from build123d import *

# Parameters (mm, degrees)
SKETCH1_R           = 31.5
SKETCH1_R_2         = 2.6
BOSS_EXTRUDE1_DEPTH = 5
SKETCH2_R           = 12.53
SKETCH2_R_2         = 9.53
BOSS_EXTRUDE2_DEPTH = 15
CUT_EXTRUDE1_START  = -7
CUT_EXTRUDE1_DEPTH  = 7
FILLET1_R           = 5
FILLET2_R           = 2
FILLET3_R           = 2


with BuildPart() as part:
    # Sketch1 → Boss-Extrude1 (new body)
    with BuildSketch(Plane.XY):
        Circle(SKETCH1_R)
        with Locations((0, 25)):
            Circle(SKETCH1_R_2, mode=Mode.SUBTRACT)
        with Locations((25, 0)):
            Circle(SKETCH1_R_2, mode=Mode.SUBTRACT)
        with Locations((0, -25)):
            Circle(SKETCH1_R_2, mode=Mode.SUBTRACT)
        with Locations((-25, 0)):
            Circle(SKETCH1_R_2, mode=Mode.SUBTRACT)
    extrude(amount=BOSS_EXTRUDE1_DEPTH)

    # Sketch2 → Boss-Extrude2 (add)
    with BuildSketch(Plane.XY.offset(5)):
        Circle(SKETCH2_R)
        Circle(SKETCH2_R_2, mode=Mode.SUBTRACT)
    extrude(amount=BOSS_EXTRUDE2_DEPTH)

    # Sketch3 → Cut-Extrude1 (cut)
    with BuildSketch(Plane.XY.offset(5).offset(CUT_EXTRUDE1_START)):
        with BuildLine():
            ThreePointArc((-14.488887394, 3.882285677), (-10.606601718, 10.606601718), (-3.882285677, 14.488887394))
            Line((-3.882285677, 14.488887394), (-8.152799921, 30.426663528))
            ThreePointArc((-8.152799921, 30.426663528), (-22.273863607, 22.273863607), (-30.426663528, 8.152799921))
            Line((-30.426663528, 8.152799921), (-14.488887394, 3.882285677))
        make_face()
        with BuildLine():
            Line((8.152799921, 30.426663528), (3.882285677, 14.488887394))
            ThreePointArc((3.882285677, 14.488887394), (10.606601718, 10.606601718), (14.488887394, 3.882285677))
            Line((14.488887394, 3.882285677), (30.426663528, 8.152799921))
            ThreePointArc((30.426663528, 8.152799921), (22.273863607, 22.273863607), (8.152799921, 30.426663528))
        make_face()
        with BuildLine():
            Line((30.426663528, -8.152799921), (14.488887394, -3.882285677))
            ThreePointArc((14.488887394, -3.882285677), (10.606601718, -10.606601718), (3.882285677, -14.488887394))
            Line((3.882285677, -14.488887394), (8.152799921, -30.426663528))
            ThreePointArc((8.152799921, -30.426663528), (22.273863607, -22.273863607), (30.426663528, -8.152799921))
        make_face()
        with BuildLine():
            Line((-8.152799921, -30.426663528), (-3.882285677, -14.488887394))
            ThreePointArc((-3.882285677, -14.488887394), (-10.606601718, -10.606601718), (-14.488887394, -3.882285677))
            Line((-14.488887394, -3.882285677), (-30.426663528, -8.152799921))
            ThreePointArc((-30.426663528, -8.152799921), (-22.273863607, -22.273863607), (-8.152799921, -30.426663528))
        make_face()
    extrude(amount=CUT_EXTRUDE1_DEPTH, mode=Mode.SUBTRACT)

    # Fillet1
    fillet1_edges = [part.edges().sort_by_distance(p)[0] for p in [
        (-8.152799921, -30.426663528, 2.5),
        (-30.426663528, -8.152799921, 2.5),
        (30.426663528, -8.152799921, 2.5),
        (8.152799921, -30.426663528, 2.5),
        (8.152799921, 30.426663528, 2.5),
        (30.426663528, 8.152799921, 2.5),
        (-30.426663528, 8.152799921, 2.5),
        (-8.152799921, 30.426663528, 2.5),
    ]]
    fillet(fillet1_edges, radius=FILLET1_R)

    # Fillet2
    fillet2_edges = [part.edges().sort_by_distance(p)[0] for p in [
        (-14.488887394, -3.882285677, 2.5),
        (-3.882285677, -14.488887394, 2.5),
        (3.882285677, -14.488887394, 2.5),
        (14.488887394, -3.882285677, 2.5),
        (14.488887394, 3.882285677, 2.5),
        (3.882285677, 14.488887394, 2.5),
        (-3.882285677, 14.488887394, 2.5),
        (-14.488887394, 3.882285677, 2.5),
    ]]
    fillet(fillet2_edges, radius=FILLET2_R)

    # Fillet3
    fillet3_edges = [part.edges().sort_by_distance(p)[0] for p in [
        (-12.53, 0, 5),
    ]]
    fillet(fillet3_edges, radius=FILLET3_R)


solid = part.part
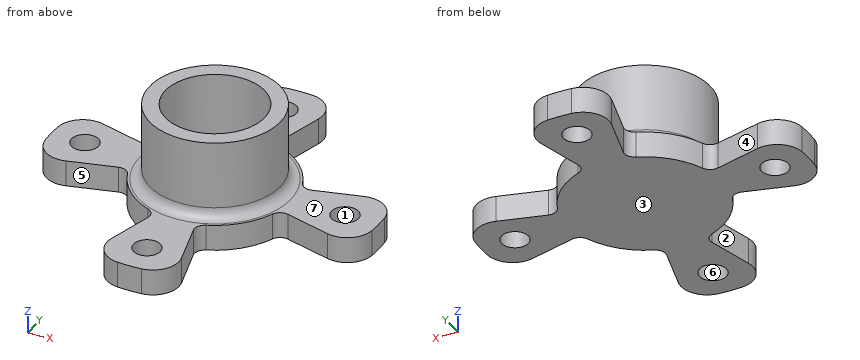
Geometry: final body of the model. Coordinates: model frame, mm. Face numbers are marked on the shaded views. A direction names the side the tool comes from. Give positions to 0.01 mm unless a question says otherwise; leave off trailing zeros. Write each loop counter-clockwise with the first axis right and the second up, starting at its lowest first coordinate (ties: lowest second). Pieces come first, ordered by that corner, then holes.
(1) Ray query, line 1 (Y direction, x = 0, z = 16.25); line 2 (Y direction, x = 0, z = 2.7); line 3 (Z direction, x = 4.5, y = 0.5). Return the intervals inside material, ascending.
(2) Cut plane A-A, the plane y = 0. Return loops of the section in (x, z).
(3) Cut plane C-C, the plane z = 3.25. Give the number of separate pieces and of enclosed holes in the cut face, then the cut area to 3 significant figures.
(4) Mould query, pull axis X, two halves, no side actions, for the marked faces 1, 2 and 3. Classes: released by +X, released by -X, zero draft, split by the parting line, or undercut.
(5) Cut plane B-B, the plane x = -24. Return loops of the section in (y, z), then the cut area to 3 significant figures.
(6) Cut plane D-D, the plane z = 17.5. Return loops of the section in (x, y), then the cut area to 3 significant figures.
(7) Access query for the marked faces 4, 5, 6 and 7. Directions: +Z, -Z, +X, -X, +Y, -Y. A direction counts if a zero-diameter tool reaches every point of the face in a straight line with its end or side. Return the directions, or none.
(8) First-contact query: P1, Ø3, axis at x = 3, y = -12.5, coming from the +Z side; P2, Ø2, axis at x = -5.5, z = 16.5, coming from the -Y side; P3, Ø4, axis at x = 0, y = 25, coming from the -Z side (3 decimals); P4, Ø12, axis at y = -7.5, z = 15, coming from the +X side. Flat tips, straight axial feed; report the tip coordinate or a pass-through.
Values follow:
1. line 1: y = -12.53 to -9.53, 9.53 to 12.53
1. line 2: y = -31.5 to -27.6, -22.4 to 22.4, 27.6 to 31.5
1. line 3: z = 0 to 5
2. outline: (-31.5, 0) - (-27.6, 0) - (-27.6, 5) - (-31.5, 5) - close; (-22.4, 0) - (22.4, 0) - (22.4, 5) - (14.53, 5) arc R2 cw to (12.53, 7) - (12.53, 20) - (9.53, 20) - (9.53, 5) - (-9.53, 5) - (-9.53, 20) - (-12.53, 20) - (-12.53, 7) arc R2 cw to (-14.53, 5) - (-22.4, 5) - close; (27.6, 0) - (31.5, 0) - (31.5, 5) - (27.6, 5) - close
3. separate pieces: 1
3. enclosed holes: 4
3. area: 1,370 mm2
4. face 1: undercut
4. face 2: released by -X
4. face 3: zero draft
5. outline: (-6.43, 0) - (-2.4, 0) - (-2.4, 5) - (-6.43, 5) - close; (2.4, 0) - (6.43, 0) - (6.43, 5) - (2.4, 5) - close
5. area: 40.3 mm2
6. outline: circle Ø25.06 at (0, 0); hole circle Ø19.06 at (0, 0)
6. area: 208 mm2
7. face 4: +Z, -Z, +Y
7. face 5: +Z, -Z, -Y
7. face 6: +Z, -Z
7. face 7: +Z
8. P1: stops at z = 20
8. P2: stops at y = -11.69
8. P3: passes through
8. P4: stops at x = 12.44
